Verification items for the finished model (mm, model axes). Round coordinates to 2 decimals unless told otherwise and drop trailing zeros. Order: outer loops, then holes, each group sorted by start corner. A loop starts at its lowest first (then second) coordinate and runs counter-clockwise, first axis right, second up. Notation, with made-up numbers: (61.5, 61) -> (68.5, 61) arc R20 cw to (68.5, 100) -> close; hole circle Ø3 at (72, 79.5). An arc over 180 degrees is marked (long way). Put each result on its own line as item: value.
from build123d import *

# Parameters (mm, degrees)
SKETCH_R    = 4
PAD_DEPTH   = 6
FILLET_R    = 3
FILLET001_R = 1


with BuildPart() as part:
    # Sketch → Pad (new body)
    with BuildSketch(Plane.XY):
        with BuildLine():
            Line((-20, 132), (-80, 26))
            Line((-80, 26), (-80, 6))
            Line((-80, 6), (-73.167603, 0))
            Line((-73.167603, 0), (-57.167603, 0))
            Line((-57.167603, 0), (-50.335206, 6))
            Line((-50.335206, 6), (50.335206, 6))
            Line((50.335206, 6), (57.167603, 0))
            Line((57.167603, 0), (73.167603, 0))
            Line((73.167603, 0), (80, 6))
            Line((80, 6), (80, 26))
            Line((80, 26), (20, 132))
            Line((20, 132), (20, 150))
            Line((4, 150), (20, 150))
            Line((4, 140), (4, 150))
            ThreePointArc((-4, 140), (0, 136), (4, 140))
            Line((-4, 150), (-4, 140))
            Line((-20, 150), (-4, 150))
            Line((-20, 132), (-20, 150))
        make_face()
        with Locations((-65.167603, 16)):
            Circle(SKETCH_R, mode=Mode.SUBTRACT)
        with Locations((65.167603, 16)):
            Circle(SKETCH_R, mode=Mode.SUBTRACT)
        Polygon((-54.799288, 29.920219), (-8, 112.59896), (8, 112.59896), (54.799288, 29.920219), (50.335206, 26), (-50.335206, 26), align=None, mode=Mode.SUBTRACT)
    extrude(amount=PAD_DEPTH)

    # Fillet
    fillet_edges = [part.edges().sort_by_distance(p)[0] for p in [
        (-20, 132, 3),
        (-80, 26, 3),
        (-80, 6, 3),
        (-73.167603, 0, 3),
        (-57.167603, 0, 3),
        (-50.335206, 6, 3),
        (50.335206, 6, 3),
        (57.167603, 0, 3),
        (73.167603, 0, 3),
        (80, 6, 3),
        (80, 26, 3),
        (20, 132, 3),
        (20, 150, 3),
        (4, 150, 3),
        (-4, 150, 3),
        (-20, 150, 3),
        (-54.799288, 29.920219, 3),
        (-8, 112.59896, 3),
        (8, 112.59896, 3),
        (54.799288, 29.920219, 3),
        (50.335206, 26, 3),
        (-50.335206, 26, 3),
    ]]
    fillet(fillet_edges, radius=FILLET_R)

    # Fillet001
    fillet001_edges = [part.edges().sort_by_distance(p)[0] for p in [
        (-50, 79, 6),
        (-31.229726, 71.559778, 6),
    ]]
    fillet(fillet001_edges, radius=FILLET001_R)


solid = part.part
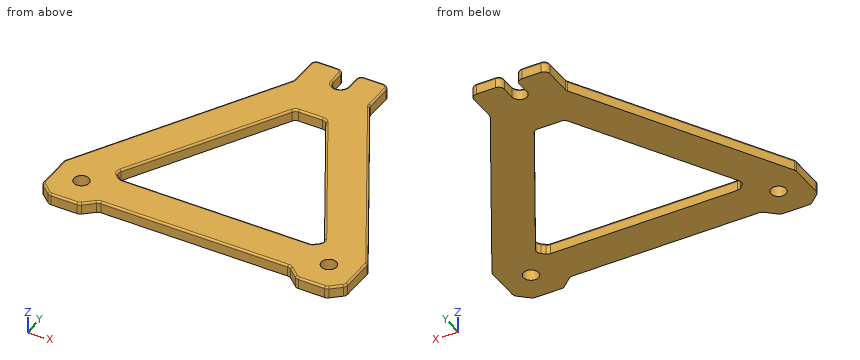
Item 1: Section check A-A on x = 0. Record the boundary of the cut face in (y, z), then the cut area to 3 significant figures.
Check sheet entries:
outline: (6, 0) -> (26, 0) -> (26, 5) arc R1 ccw to (25, 6) -> (7, 6) arc R1 ccw to (6, 5) -> close; (112.6, 0) -> (136, 0) -> (136, 5) arc R1 ccw to (135, 6) -> (113.6, 6) arc R1 ccw to (112.6, 5) -> close
area: 260 mm^2
Item 2: Section check C-C on z = 2.5. State how many separate pieces and enclosed holes the cut face has, then the cut area to 3 significant figures.
Check sheet entries:
separate pieces: 1
enclosed holes: 3
area: 8,980 mm^2
Item 3: Gauge pin test, flat ends, axial feed: pin 1 Ø1.5 at (y, z) = (143, 3.5) entering from -X; pin 2 Ø9 at (x, y) = (-65.17, 16) entering from +Z; pin 3 Ø2.5 at (y, z) = (140, 3) entering from +X; pin 4 Ø1.5 at (x, z) = (-44.5, 2) entering from +Y. Record the tip position at first contact, or that the pin passes through.
Check sheet entries:
pin 1: stops at x = -20
pin 2: stops at z = 6
pin 3: stops at x = 20
pin 4: stops at y = 90.04
Item 4: Material ranges on L1, parallel to Y at x = 33, z = 4; L2, parallel to Y at x = 61.5, z = 3.75; L3, parallel to X at y = 86, z = 1, recorded low to high. Write a range as [from, to].
Check sheet entries:
L1: y = [6, 26], [68.43, 109.03]
L2: y = [0, 14.4], [17.6, 58.68]
L3: x = [-46.04, -23.06], [23.06, 46.04]
Item 5: Section check B-B on y = 16. Record the boundary of the cut face in (x, z).
Check sheet entries:
outline: (-80, 0) -> (-69.17, 0) -> (-69.17, 6) -> (-79, 6) arc R1 ccw to (-80, 5) -> close; (-61.17, 0) -> (61.17, 0) -> (61.17, 6) -> (-61.17, 6) -> close; (69.17, 0) -> (80, 0) -> (80, 5) arc R1 ccw to (79, 6) -> (69.17, 6) -> close
